For this review, take the finished solid that the model builds, in its own axes (mm). Face numbers are marked on the shaded views. A direction names the side the tool comes from. Round coordinates to 2 decimals unless told otherwise and drop trailing zeros. Order: outer loops, then holes, each group sorted by start corner. A loop starts at its lowest first (then second) coordinate and runs counter-clockwise, first axis right, second up. Notation, with made-up numbers: (15.25, -38) -> (37.25, -38) arc R17 ccw to (37.25, -10) -> close; hole circle Ø3 at (-1, 18). An arc over 180 degrees is marked (long way). Answer in a Markdown table with one row per item.
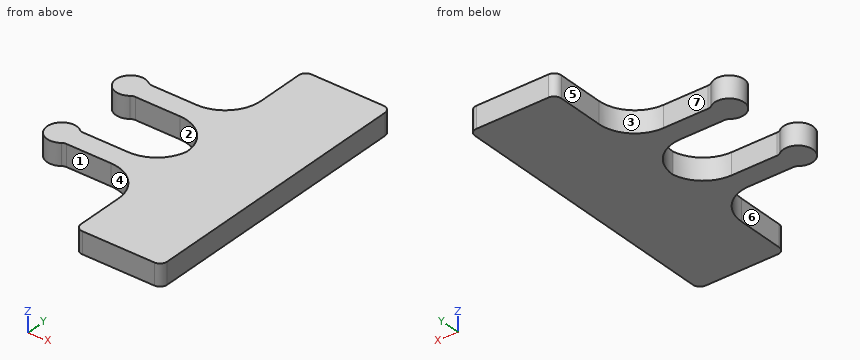
Autodesk Inventor part; units mm, degrees
ref_plane "Plan YZ" through (0, 0, 0) normal (1, 0, 0) x (0, 1, 0)
ref_plane "Plan XZ" through (0, 0, 0) normal (0, 1, 0) x (-1, 0, 0)
ref_plane "Plan XY" through (0, 0, 0) normal (0, 0, 1) x (1, 0, 0)
sketch "Esquisse1" plane through (0, 0, 0) normal (0, 0, 1) x (1, 0, 0)
  arc A0 (-11.55, 1.45) -> (-11.55, -1.45) centre (-13, 0) ccw
  line L0 (-13, 0) -> (-11.55, -1.45) construction
  line L1 (-13, 0) -> (-10.9494, 0) construction
  line L2 (-13, 0) -> (-11.55, 1.45) construction
  line L3 (-11.55, 1.45) -> (0, 1.45)
  line L4 (-11.55, -1.45) -> (0, -1.45)
  line L5 (0, -34) -> (0, 22) construction
  line L6 (-20.4607, 0) -> (17.4101, 0) construction
  line L7 (-5, -6) -> (5, -6) construction
  arc A1 (-11.55, -10.55) -> (-11.55, -13.45) centre (-13, -12) ccw
  line L8 (-11.55, -13.45) -> (0, -13.45)
  line L9 (-11.55, -10.55) -> (0, -10.55)
  line L10 (0, -26) -> (12, -26)
  line L11 (12, -26) -> (12, 14)
  line L12 (12, 14) -> (0, 14)
  line L13 (0, 14) -> (0, -26)
  line L14 (0, -26) -> (12, 14) construction
  line L15 (12, -26) -> (0, 14) construction
  point P0 (0, 0)
  point P1 (0, -6)
  point P2 (6, -6)
  point P3 (0, -13.45)
  dimension "d0" = 45
  dimension "d1" = 90
  dimension "d3" = 13
  dimension "d7" = 2.9
  dimension "d8" = 10
  dimension "d9" = 6
  dimension "d10" = 12
  dimension "d11" = 40
extrude "Extrusion2" add sketch "Esquisse1" along normal blind 3
fillet "Congé2" radius 0.95 4 edges at (-11.55, -13.45, 1.5) (-11.55, -10.55, 1.5) (-11.55, -1.45, 1.5) (-11.55, 1.45, 1.5)
fillet "Congé3" radius 1 4 edges at (0, -26, 1.5) (12, -26, 1.5) (0, 14, 1.5) (12, 14, 1.5)
fillet "Congé4" radius 5 4 edges at (0, -13.45, 1.5) (0, -1.45, 1.5) (0, -10.55, 1.5) (0, 1.45, 1.5)
properties part number "T2601_Conn" material "."
Q1. Clearance check with flat-ended pins moving along their axes: pin 1 Ø0.9 at (y, z) = (-20, 2) entering from -X; pin 2 Ø1.5 at (x, z) = (-8.5, 1.5) entering from -Y; pin 3 Ø0.9 at (x, z) = (-9, 1) entering from +Y. State where each tip first meets the part, or that it passes through.
Answer key:
| item | result |
|---|---|
| pin 1 | stops at x = 0 |
| pin 2 | stops at y = -13.45 |
| pin 3 | stops at y = 1.45 |
Q2. Tool access review of the marked faces 4, 5, 6 and 7: name each direction out of +Z, -Z, +X, -X, +Y, -Y from which nothing blocks a thin tool from reaching the whole face with its end or side.
Answer key:
| item | result |
|---|---|
| face 4 | +Z, -Z, -Y |
| face 5 | +Z, -Z, -X, +Y |
| face 6 | +Z, -Z, -X, -Y |
| face 7 | +Z, -Z, +Y |
Q3. Take a section at D-D, the plane y = 3. Write out the cut boundary in (x, z).
Answer key:
| item | result |
|---|---|
| outline | (-1.38, 0) -> (12, 0) -> (12, 3) -> (-1.38, 3) -> close |
Q4. Take a section at A-A, the plane x = -13. Write out the cut boundary in (y, z), then the cut area to 3 significant figures.
Answer key:
| item | result |
|---|---|
| outline | (-14.05, 0) -> (-9.95, 0) -> (-9.95, 3) -> (-14.05, 3) -> close; (-2.05, 0) -> (2.05, 0) -> (2.05, 3) -> (-2.05, 3) -> close |
| area | 24.6 mm^2 |
Q5. Take a section at B-B, the plane z = 1.1. Write out the cut boundary in (x, y), then the cut area to 3 significant figures.
Answer key:
| item | result |
|---|---|
| outline | (-11.77, -13.64) arc R0.95 cw to (-11.2, -13.45) -> (-5, -13.45) arc R5 cw to (0, -18.45) -> (0, -25) arc R1 ccw to (1, -26) -> (11, -26) arc R1 ccw to (12, -25) -> (12, 13) arc R1 ccw to (11, 14) -> (1, 14) arc R1 ccw to (0, 13) -> (0, 6.45) arc R5 cw to (-5, 1.45) -> (-11.2, 1.45) arc R0.95 cw to (-11.77, 1.64) arc R2.05 ccw (long way) to (-11.77, -1.64) arc R0.95 cw to (-11.2, -1.45) -> (-5, -1.45) arc R5 cw to (0, -6.45) arc R5 cw to (-4.92, -10.55) -> (-11.2, -10.55) arc R0.95 cw to (-11.77, -10.36) arc R2.05 ccw (long way) to start |
| area | 591 mm^2 |
Q6. Take a section at C-C, the plane y = -21.5. Write out the cut boundary in (x, z), then the cut area to 3 significant figures.
Answer key:
| item | result |
|---|---|
| outline | (0, 0) -> (12, 0) -> (12, 3) -> (0, 3) -> close |
| area | 36.0 mm^2 |
Q7. The part is to be moulded in two halves that separate along Y. For the marked faces 1, 2 and 3, say which applies: +Y half, -Y half, draft (parallel to the pull), parting line (faces both ways), or undercut.
Answer key:
| item | result |
|---|---|
| face 1 | -Y half |
| face 2 | undercut |
| face 3 | +Y half |
Q8. To check wall thickness, follow probe 1 along Y at (x, z) = (-8.5, 1.85); probe 2 along X at (y, z) = (-23, 1.3); probe 3 along Y at (x, z) = (-4, 1.9). State the ranges of each line that lie inside material, in increasing order.
Answer key:
| item | result |
|---|---|
| probe 1 | y = -13.45 to -10.55, -1.45 to 1.45 |
| probe 2 | x = 0 to 12 |
| probe 3 | y = -13.55 to -10.46, -1.55 to 1.55 |
